from build123d import *

# Parameters (mm, degrees)
CUT_EXTRUDE1_REACH = 86.593
SKETCH2_W          = 13.839504146
SKETCH2_H          = 1.5875
FILLET1_R          = 3.175


with BuildPart() as part:
    # Sketch1 → Revolve1 (revolve)
    with BuildSketch(Plane.XY, mode=Mode.PRIVATE) as revolve1_sk:
        Polygon((0, 9.525), (81.5594, 9.525), (81.5594, 12.7), (78.3844, 12.7), (78.3844, 11.9126), (76.2, 11.9126), (76.2, 12.7), (2.54, 12.7), (2.54, 15.875), (0, 15.875), align=None)
    revolve(revolve1_sk.sketch.rotate(Axis((0, 0, 0), (1, 0, 0)), 90), axis=Axis((0, 0, 0), (1, 0, 0)))

    # Sketch2 → Cut-Extrude1 (cut, up to next)
    with BuildSketch(Plane.ZY, mode=Mode.PRIVATE) as cut_extrude1_sk1:
        with Locations((0, 15.08125)):
            Rectangle(SKETCH2_W, SKETCH2_H)
    cut_extrude1_tool1 = extrude(cut_extrude1_sk1.sketch, amount=-CUT_EXTRUDE1_REACH, mode=Mode.PRIVATE) & part.part
    # Sketch2 → Cut-Extrude1 (cut, up to next)
    with BuildSketch(Plane.ZY, mode=Mode.PRIVATE) as cut_extrude1_sk2:
        with Locations((0, -15.08125)):
            Rectangle(SKETCH2_W, SKETCH2_H)
    cut_extrude1_tool2 = extrude(cut_extrude1_sk2.sketch, amount=-CUT_EXTRUDE1_REACH, mode=Mode.PRIVATE) & part.part
    add(cut_extrude1_tool1.solids().sort_by_distance((0, 15.08125, 0))[0], mode=Mode.SUBTRACT)
    add(cut_extrude1_tool2.solids().sort_by_distance((0, -15.08125, 0))[0], mode=Mode.SUBTRACT)

    # Fillet1
    fillet1_edges = [part.edges().sort_by_distance(p)[0] for p in [
        (1.27, 14.2875, -6.919752073),
        (1.27, 14.2875, 6.919752073),
        (1.27, -14.2875, -6.919752073),
        (1.27, -14.2875, 6.919752073),
    ]]
    fillet(fillet1_edges, radius=FILLET1_R)


solid = part.part
CAD build for the part. Positions are in the model's coordinates, mm. A direction names the side the tool comes from. Round coordinates to 2 decimals unless told otherwise and drop trailing zeros. Order: outer loops, then holes, each group sorted by start corner. A loop starts at its lowest first (then second) coordinate and runs counter-clockwise, first axis right, second up. Notation, with made-up numbers: (-40, -23) -> (-18, -23) arc R19 ccw to (-18, -4) -> close; hole circle Ø8 at (16, 13). An arc over 180 degrees is marked (long way). Write item = value, one per line. Start each with the question number.
(1) Cut at C-C, the plane x = 22. List the corners of the cut face in (y, z) (3 decimals), then the cut area to 3 significant figures.
(2) Pull direction X, two halves, no side cores. Call faces 1 (the flat face through (0, -7, -7)), 2 (the cylindrical face through (41.35, 9.3, -2.06)), 3 (the cylindrical face through (77.28, 7.25, -9.45)): released by +X, released by -X, zero draft, split by the parting line, or undercut.
(3) Probe line 1 (Y direction, x = 64, z = 0) (3 decimals); line 2 (Z direction, x = 62, y = -6); line 3 (Z direction, x = 27, y = 3). List the from-to ranges inside material, lowest first. Write a range as [from, to].
(4) Which spindle directions (+Z, -Z, +X, -X, +Y, -Y) get a long thin tool onto all of the face, cutting with end or side? Do faces 4 (the cylindrical face through (1.252, -0.237, -15.873)), 5 (the cylindrical face through (38.9, 7.7, -10.1)). Say none if no direction does.
(5) Cut at B-B, the plane z = 0. List the corners of the cut face in (x, y) (1 decimal).
(6) Cut at A-A, the plane y = 0. List the corners of the cut face in (x, z) (3 decimals), then the cut area to 3 significant figures.
(7) Cut at D-D, the plane y = -11. List the corners of the cut face in (x, z).
(8) Pin check, flat tips, straight feed: P1, Ø1, axis at x = 19, z = -5.5, coming from the -Y side; P2, Ø2, axis at x = 16, z = -4.5, coming from the -Y side; P3, Ø15, axis at y = 0, z = 0, coming from the +X side; P4, Ø6, axis at x = 16, y = -5, coming from the -Z side. Stop position of each tip, or through.
Model answer:
q1.outline = circle Ø25.4 at (0, 0); hole circle Ø19.05 at (0, 0)
q1.area = 222 mm2
q2.face_1 = released by -X
q2.face_2 = zero draft
q2.face_3 = undercut
q3.line_1 = [-12.7, -9.525], [9.525, 12.7]
q3.line_2 = [-11.19, -7.4], [7.4, 11.19]
q3.line_3 = [-12.34, -9.04], [9.04, 12.34]
q4.face_4 = -Z, +X, -X
q4.face_5 = +X
q5.outline = (0, -14.3) -> (2.5, -14.3) -> (2.5, -12.7) -> (76.2, -12.7) -> (76.2, -11.9) -> (78.4, -11.9) -> (78.4, -12.7) -> (81.6, -12.7) -> (81.6, -9.5) -> (0, -9.5) -> close; (0, 9.5) -> (81.6, 9.5) -> (81.6, 12.7) -> (78.4, 12.7) -> (78.4, 11.9) -> (76.2, 11.9) -> (76.2, 12.7) -> (2.5, 12.7) -> (2.5, 14.3) -> (0, 14.3) -> close
q6.outline = (0, -15.875) -> (2.54, -15.875) -> (2.54, -12.7) -> (76.2, -12.7) -> (76.2, -11.913) -> (78.384, -11.913) -> (78.384, -12.7) -> (81.559, -12.7) -> (81.559, -9.525) -> (0, -9.525) -> close; (0, 9.525) -> (81.559, 9.525) -> (81.559, 12.7) -> (78.384, 12.7) -> (78.384, 11.913) -> (76.2, 11.913) -> (76.2, 12.7) -> (2.54, 12.7) -> (2.54, 15.875) -> (0, 15.875) -> close
q6.area = 531 mm2
q7.outline = (0, -11.45) -> (2.54, -11.45) -> (2.54, -6.35) -> (76.2, -6.35) -> (76.2, -4.57) -> (78.38, -4.57) -> (78.38, -6.35) -> (81.56, -6.35) -> (81.56, 6.35) -> (78.38, 6.35) -> (78.38, 4.57) -> (76.2, 4.57) -> (76.2, 6.35) -> (2.54, 6.35) -> (2.54, 11.45) -> (0, 11.45) -> close
q8.P1 = -11.67
q8.P2 = -12.21
q8.P3 = through
q8.P4 = -12.54
